Input: part model. Units: mm. Frame: model coordinates. A direction names the side the tool comes from. Coordinates: 2 decimals unless noted, no trailing zeros. Write each loop counter-clockwise with the first axis right and the second up, starting at its lowest first coordinate (ties: lowest second). Pieces come first, ordered by that corner, then holes. Notation, with made-up numbers: M 83.25,78.5 L 119.25,78.5 A13 ccw 119.25,82.5 Z; hole C -14,71.5 d6. An arc over 180 degrees is marked long. Use one line per item in the form item = value.
from build123d import *

# Parameters (mm, degrees)
F0_W      = 50
F0_H      = 60
F1_DEPTH  = 5
F4_START  = 2
F3_W      = 58
F3_H      = 60
F4_DEPTH  = 3
F2_W      = 45.5
F2_H      = 45.5
F5_DEPTH  = 3
F7_START  = 1.5
F6_W      = 20
F6_H      = 30
F7_DEPTH  = 1.5
F8_W      = 2
F8_H      = 56
F9_DEPTH  = 25
F10_R     = 2
F11_W     = 5
F11_H     = 1.5
F12_DEPTH = 2
F13_SIZE  = 1.5


with BuildPart() as f1:
    # F0 (on Top) → F1 (new body)
    with BuildSketch(Plane.XY):
        Rectangle(F0_W, F0_H)
    extrude(amount=F1_DEPTH)

    # F3 (on Top) → F4 (join)
    with BuildSketch(Plane.XY.offset(F4_START)):
        Rectangle(F3_W, F3_H)
    extrude(amount=F4_DEPTH)

    # F2 (on Top) → F5 (cut)
    with BuildSketch(Plane.XY):
        Rectangle(F2_W, F2_H)
    extrude(amount=F5_DEPTH, mode=Mode.SUBTRACT)

    # F6 (on Top) → F7 (cut)
    with BuildSketch(Plane.XY.offset(F7_START)):
        with Locations((0, -15)):
            Rectangle(F6_W, F6_H)
    extrude(amount=F7_DEPTH, mode=Mode.SUBTRACT)

    # F8 (on Top) → F9 (cut)
    with BuildSketch(Plane.XY):
        with Locations((-26, 0)):
            Rectangle(F8_W, F8_H)
        with Locations((26, 0)):
            Rectangle(F8_W, F8_H)
    extrude(amount=F9_DEPTH, mode=Mode.SUBTRACT)

    # F10
    f10_edges = [f1.edges().sort_by_distance(p)[0] for p in [
        (29, -30, 3.5),
        (-29, -30, 3.5),
        (-29, 30, 3.5),
        (29, 30, 3.5),
    ]]
    fillet(f10_edges, radius=F10_R)

    # F11 (on Top) → F12 (join)
    with BuildSketch(Plane.XY):
        with Locations((-14.75, -30.75)):
            Rectangle(F11_W, F11_H)
        with Locations((14.75, -30.75)):
            Rectangle(F11_W, F11_H)
        with Locations((14.75, 30.75)):
            Rectangle(F11_W, F11_H)
        with Locations((-14.75, 30.75)):
            Rectangle(F11_W, F11_H)
    extrude(amount=F12_DEPTH)

    # F13
    f13_edges = [f1.edges().sort_by_distance(p)[0] for p in [
        (-14.75, -31.5, 0),
        (14.75, -31.5, 0),
        (14.75, 31.5, 0),
        (-14.75, 31.5, 0),
    ]]
    chamfer(f13_edges, length=F13_SIZE)


solid = f1.part
(1) Set-up query: faces 1 (the flat face through (17.25, 30.6, 1.2)), 2 (the flat face through (15, -31, 2)), 3 (the flat face through (-26, -28, 3)), 4 (the flat face through (0, -26, 1.5)). Return all of +Z, -Z, +X, -X, +Y, -Y with unobstructed straight access to the full face (end or side cutting, diameter ignored); none if empty.
Computed:
face_1 = +Z, -Z, +X, +Y
face_2 = +Z, +X, -X, -Y
face_3 = +Z, -Z
face_4 = -Y
(2) Section query A-A on y = 7. Return the cut outline in (x, z), plus the area to 4 significant figures.
Computed:
outline = M -29,2 L -27,2 L -27,5 L -29,5 Z; M -25,0 L -22.75,0 L -22.75,3 L 22.75,3 L 22.75,0 L 25,0 L 25,5 L -25,5 Z; M 27,2 L 29,2 L 29,5 L 27,5 Z
area = 125.5 mm^2
(3) First-contact query: pin 1 Ø4.5 at (x, y) = (27.5, 14) entering from -Z; pin 2 Ø1.5 at (x, z) = (8, 1.5) entering from +Y; pin 3 Ø13.5 at (x, y) = (4, 0.5) entering from -Z. Flat tips, straight axial feed; report the tip coordinate or a pass-through.
Computed:
pin_1 = 2
pin_2 = 30
pin_3 = 3
(4) Pull-direction query (Y, two-part tool) for faces 5 (the flat face through (-15, 31, 1)), 6 (the flat face through (-26, 28, 3)), 7 (the flat face through (-12.25, 30.6, 1.2)), 8 (the flat face through (0, -22.75, 1)); classes: pulls with the +Y half, pulls with the -Y half, needs draft (parallel to the pull), parting line crosses it, or undercut.
Computed:
face_5 = pulls with the +Y half
face_6 = undercut
face_7 = needs draft
face_8 = undercut
(5) Section query D-D on x = 16.5. Return the cut outline in (y, z), plus the area to 3 significant figures.
Computed:
outline = M -31.5,1.5 L -30,0 L -22.75,0 L -22.75,3 L 22.75,3 L 22.75,0 L 30,0 L 31.5,1.5 L 31.5,2 L 30,2 L 30,5 L -30,5 L -30,2 L -31.5,2 Z
area = 167 mm^2
(6) Line query: probe 1 along X at (y, z) = (-21, 4.1); probe 2 along X at (y, z) = (-9.5, 0.3); probe 3 along Y at (x, z) = (-9, 0.35). Output: solid intervals per line, ascending.
Computed:
probe_1 = -29 to -27, -25 to 25, 27 to 29
probe_2 = -25 to -22.75, 22.75 to 25
probe_3 = -30 to -22.75, 22.75 to 30
(7) Section query C-C on z = 3.75. Return the cut outline in (x, y).
Computed:
outline = M -29,-28 A2 ccw -27,-30 L 27,-30 A2 ccw 29,-28 L 29,28 A2 ccw 27,30 L -27,30 A2 ccw -29,28 Z; hole M -27,-28 L -25,-28 L -25,28 L -27,28 Z; hole M 25,-28 L 27,-28 L 27,28 L 25,28 Z
(8) Section query B-B on x = -3.5. Return the cut outline in (y, z).
Computed:
outline = M -30,0 L -22.75,0 L -22.75,1.5 L -30,1.5 Z; M -30,3 L 22.75,3 L 22.75,0 L 30,0 L 30,5 L -30,5 Z
